```python
from build123d import *

# Parameters (mm, degrees)
SKETCH_R     = 1.5
PAD_DEPTH    = 25.2
CHAMFER_SIZE = 0.25


with BuildPart() as part:
    # Sketch → Pad (new body)
    with BuildSketch(Plane.XY):
        Polygon((2.85, 0), (1.425, 2.468172), (-1.425, 2.468172), (-2.85, 0), (-1.425, -2.468172), (1.425, -2.468172), align=None)
        Circle(SKETCH_R, mode=Mode.SUBTRACT)
    extrude(amount=PAD_DEPTH)

    # Chamfer
    chamfer_edges = [part.edges().sort_by_distance(p)[0] for p in [
        (2.1375, 1.234086, 0),
        (0, 2.468172, 0),
        (-2.1375, 1.234086, 0),
        (-2.1375, -1.234086, 0),
        (0, -2.468172, 0),
        (2.1375, -1.234086, 0),
        (-1.5, 0, 0),
        (2.1375, 1.234086, 25.2),
        (0, 2.468172, 25.2),
        (-2.1375, 1.234086, 25.2),
        (-2.1375, -1.234086, 25.2),
        (0, -2.468172, 25.2),
        (2.1375, -1.234086, 25.2),
        (-1.5, 0, 25.2),
    ]]
    chamfer(chamfer_edges, length=CHAMFER_SIZE)


solid = part.part
```
Can you work these out from the model? Positions are in its coordinate system, mm. Give positions to 0.01 mm unless a question says otherwise; leave off trailing zeros. Order: outer loops, then holes, each group sorted by start corner. A loop starts at its lowest first (then second) coordinate and runs counter-clockwise, first axis right, second up. Notation, with made-up numbers: (12.25, 29.5) - (54.25, 29.5) arc R16 cw to (54.25, 48.5) - close; hole circle Ø10 at (16, 48.25). An arc over 180 degrees is marked (long way). Use a Markdown table: item, result. Add a question column.
Q1. Please list where these lines run through material, in increasing order: line 1 along Y through (x, z) = (0, 7.25); line 2 along X through (y, z) = (1.3, 7.75); line 3 along X through (y, z) = (-1.25, 22.75).
Q2. I'm going to push flat-ended pins straight in: pin 1 (1 mm diameter, centred on y = -1.5, z = 20, fed in from -X); pin 2 (2 mm diameter, centred on x = -1, y = 0, fed in from +Z). Where does each tip first touch, or does it pass through?
Q3. If we section it at A-A on z = 12.5: Write out the boundary of the cut face in (x, y) (3 decimals), plus the area to 3 significant figures.
Q4. If we section it at B-B on x = 0: Write out the boundary of the cut face in (y, z), plus the area to 3 significant figures.
Answers follow:
| question | item | result |
|---|---|---|
| 1 | line 1 | y = -2.47 to -1.5, 1.5 to 2.47 |
| 1 | line 2 | x = -2.1 to -0.75, 0.75 to 2.1 |
| 1 | line 3 | x = -2.13 to -0.83, 0.83 to 2.13 |
| 2 | pin 1 | stops at x = -2.27 |
| 2 | pin 2 | stops at z = 25.2 |
| 3 | outline | (-2.85, 0) - (-1.425, -2.468) - (1.425, -2.468) - (2.85, 0) - (1.425, 2.468) - (-1.425, 2.468) - close; hole circle Ø3 at (0, 0) |
| 3 | area | 14.0 mm^2 |
| 4 | outline | (-2.47, 0.25) - (-2.22, 0) - (-1.75, 0) - (-1.5, 0.25) - (-1.5, 24.95) - (-1.75, 25.2) - (-2.22, 25.2) - (-2.47, 24.95) - close; (1.5, 0.25) - (1.75, 0) - (2.22, 0) - (2.47, 0.25) - (2.47, 24.95) - (2.22, 25.2) - (1.75, 25.2) - (1.5, 24.95) - close |
| 4 | area | 48.5 mm^2 |
